Autodesk Inventor part; units mm, degrees
ref_plane "YZ Plane" through (0, 0, 0) normal (1, 0, 0) x (0, 1, 0)
ref_plane "XZ Plane" through (0, 0, 0) normal (0, 1, 0) x (-1, 0, 0)
ref_plane "XY Plane" through (0, 0, 0) normal (0, 0, 1) x (1, 0, 0)
sketch "Boceto1" plane through (0, 0, 0) normal (0, 0, 1) x (1, 0, 0)
  line L0 (0, 0) -> (8.25, 0)
  line L1 (-10.5, 2.8) -> (10.5, 2.8) construction
  line L2 (-7.75, 5.6) -> (7.75, 5.6) construction
  line L3 (10.5, 2.8) -> (8.25, 0)
  line L4 (7.75, 5.6) -> (10.5, 2.8)
  line L5 (7.75, 5.6) -> (7.75, 8.4)
  line L6 (7.75, 8.4) -> (10.55, 8.4)
  line L7 (11.95, 10.9) -> (10.55, 8.4)
  line L8 (11.95, 10.9) -> (11.95, 31.9)
  line L9 (11.95, 10.9) -> (32.95, 10.9) construction
  line L10 (9.4, 39.9) -> (11.95, 31.9)
  line L11 (9.4, 39.9) -> (9.75, 39.9) construction
  line L12 (2.95, 40.25) -> (5.95, 40.25) construction
  line L13 (0, 43.25) -> (-0.05, 43.25)
  line L14 (-3.05, 43.25) -> (-0.05, 43.25) construction
  line L15 (-0.05, 43.25) -> (-0.05, 40.25)
  line L16 (-0.05, 40.25) -> (7.95, 40.25)
  line L17 (7.95, 40.25) -> (9.4, 39.9)
  line L18 (0, 0) -> (-8.25, 0)
  line L19 (-10.5, 2.8) -> (-8.25, 0)
  line L20 (-7.75, 5.6) -> (-10.5, 2.8)
  line L21 (-7.75, 5.6) -> (-7.75, 8.4)
  line L22 (-7.75, 8.4) -> (-10.6, 8.4)
  line L23 (-12, 10.9) -> (-10.6, 8.4)
  line L24 (-12, 10.9) -> (-12, 31.9)
  line L25 (-11, 39.9) -> (-12, 31.9)
  line L26 (-11, 39.9) -> (-11.35, 39.9) construction
  line L27 (0, 43.25) -> (-1.5, 43.25)
  line L28 (-1.55, 43.25) -> (-1.55, 40.25)
  line L29 (-1.55, 40.25) -> (-9.55, 40.25)
  line L30 (-9.55, 40.25) -> (-11, 39.9)
  line L31 (-3.5, 43.25) -> (-1.5, 43.25) construction
  line L32 (0, 43.25) -> (-15, 43.25)
  line L33 (-17, 41.25) -> (-17, 15.25)
  line L34 (-17, 15.25) -> (-12, 15.25)
  line L35 (-17, 15.25) -> (-17, -10.75)
  line L36 (-15, -12.75) -> (0, -12.75)
  line L37 (16.95, 41.25) -> (16.95, 15.25)
  line L38 (16.95, 15.25) -> (11.9, 15.25)
  line L39 (16.95, 15.25) -> (16.95, -10.75)
  line L40 (14.95, -12.75) -> (0, -12.75)
  line L41 (14.95, 43.25) -> (-0.05, 43.25)
  arc A0 (-15, 43.25) -> (-17, 41.25) centre (-15, 41.25) ccw
  arc A1 (16.95, 41.25) -> (14.95, 43.25) centre (14.95, 41.25) ccw
  arc A2 (14.95, -12.75) -> (16.95, -10.75) centre (14.95, -10.75) ccw
  arc A3 (-17, -10.75) -> (-15, -12.75) centre (-15, -10.75) ccw
  point P0 (-5.95, 40.25)
  point P1 (-0.05, 43.25)
  point P2 (-17, 43.25)
  point P3 (16.95, 43.25)
  point P4 (-17, -12.75)
  point P5 (16.95, -12.75)
  point P6 (11.95, 15.25)
  point P7 (-1.55, 43.25)
  dimension "d40" = 2.8
  dimension "d45" = 90
  dimension "d52" = 8.25
  dimension "d53" = 2.8
  dimension "d54" = 2.8
  dimension "d61" = 3
  dimension "d63" = 3
  dimension "d65" = 8
  dimension "d71" = 17
  dimension "d73" = 28
  dimension "d74" = 28
  dimension "d79" = 17
  dimension "d80" = 5
  dimension "d81" = 5
  dimension "d82" = 2
extrude "Extrusión2" add sketch "Boceto1" against normal blind 5 contours L8 L10 L17 L16 L15 L13 L41 A1 L37 L38 | L34 L33 A0 L32 L28 L29 L30 L25 L24
extrude "Extrusión3" add sketch "Boceto1" against normal blind 75 contours L0 L3 L4 L5 L6 L7 L8 L38 L39 A2 L40 L36 A3 L35 L34 L24 L23 L22 L21 L20 L19 L18
properties part number "CaseV1"
Geometry: final body of the model. Coordinates: model frame, mm. A direction names the side the tool comes from. Coordinates: 2 decimals unless noted, no trailing zeros. Order: outer loops, then holes, each group sorted by start corner. A loop starts at its lowest first (then second) coordinate and runs counter-clockwise, first axis right, second up. Notation, with made-up numbers: (16, -10.75) -> (34, -10.75) arc R15 ccw to (34, 13.25) -> close; hole circle Ø8 at (72, -36). An arc over 180 degrees is marked (long way). Write item = value, one per line.
(1) Cut plane A-A on x = 1. Return loops of the section in (y, z), plus the area to 3 significant figures.
Solved:
outline = (-12.75, -75) -> (0, -75) -> (0, 0) -> (-12.75, 0) -> close; (40.25, -5) -> (43.25, -5) -> (43.25, 0) -> (40.25, 0) -> close
area = 971 mm²
(2) Pin query (flat end, axial travel): pin 1 Ø13.5 at (x, y) = (8.5, 23.5) entering from -Z; pin 2 Ø1.5 at (x, z) = (-14, -42) entering from +Y; pin 3 Ø12 at (x, y) = (-8, 5) entering from +Z; pin 4 Ø2 at (x, z) = (9, -39.5) entering from +Y. Return the tip coordinate at first contact, or that it passes through.
Solved:
pin_1 = -5
pin_2 = 15.25
pin_3 = 0
pin_4 = 8.4
(3) Line query: line 1 (X direction, y = 11, z = -55.5); line 2 (X direction, y = 8, z = -50.5); line 3 (Y direction, x = 13, z = -60.5). Output: solid intervals per line, ascending.
Solved:
line_1 = -17 to -12, 11.95 to 16.95
line_2 = -17 to -7.75, 7.75 to 16.95
line_3 = -12.75 to 15.25
(4) Cut plane C-C on z = -22.5. Return loops of the section in (x, y), plus the area to 3 significant figures.
Solved:
outline = (-17, -10.75) arc R2 ccw to (-15, -12.75) -> (14.95, -12.75) arc R2 ccw to (16.95, -10.75) -> (16.95, 15.25) -> (11.95, 15.25) -> (11.95, 10.9) -> (10.55, 8.4) -> (7.75, 8.4) -> (7.75, 5.6) -> (10.5, 2.8) -> (8.25, 0) -> (-8.25, 0) -> (-10.5, 2.8) -> (-7.75, 5.6) -> (-7.75, 8.4) -> (-10.6, 8.4) -> (-12, 10.9) -> (-12, 15.25) -> (-17, 15.25) -> close
area = 641 mm²
(5) Pull-direction query (X, two-part tool) for faces 1 (the flat face through (-11.493, 35.956, -2.465)), 2 (the flat face through (-9.39, 1.42, -36.98)), 3 (the flat face through (-8, 43.25, -2)), 4 (the cylindrical face through (-16.43, -12.15, -36.98)); classes: pulls with the +X half, pulls with the -X half, needs draft (parallel to the pull), parting line crosses it, or undercut.
Solved:
face_1 = undercut
face_2 = undercut
face_3 = needs draft
face_4 = pulls with the -X half
(6) Cut plane B-B on y = 7.5. Return loops of the section in (x, z), plus the area to 3 significant figures.
Solved:
outline = (-17, -75) -> (-7.75, -75) -> (-7.75, 0) -> (-17, 0) -> close; (7.75, -75) -> (16.95, -75) -> (16.95, 0) -> (7.75, 0) -> close
area = 1,380 mm²
(7) Access query for faces 5 (the flat face through (9.39, 1.42, -36.98)), 6 (the flat face through (-17, 4, -37)), 7 (the flat face through (14, 15.25, -40)), 8 (the flat face through (-0.05, 42, -2)). Directions: +Z, -Z, +X, -X, +Y, -Y. A direction counts if a zero-diameter tool reaches every point of the face in a straight line with its end or side. Return the directions, or none.
Solved:
face_5 = +Z, -Z
face_6 = +Z, -Z, -X, +Y, -Y
face_7 = -Z, +X, -X, +Y
face_8 = +Z, -Z, +Y
